Part model, mm, in its own coordinate system. A direction names the side the tool comes from. Round coordinates to 2 decimals unless told otherwise and drop trailing zeros. Write each loop counter-clockwise with the first axis right and the second up, starting at its lowest first coordinate (ties: lowest second). Pieces come first, ordered by that corner, then holes. Notation, with made-up numbers: M 60,39 L 66,39 A33 ccw 66,72 Z; hole C -20.5,89 d8. An arc over 180 degrees is marked long. Use one line per item in the form item = value. Start each with the question number.
Item 1: Mould opens along Y. For faces 5 (the face through (-15, 0, 20)), 6 (the face through (20, 10, 20)), 7 (the face through (14.141, 2.797, 20.07)) say: +Y half, -Y half, draft (parallel to the pull), parting line (faces both ways), or undercut.
Item 2: Cut at D-D, the plane z = 34. Give the cut face in (x, y), then the cut area to 3 significant figures.
Item 3: Flat gauge pins, fed straight in: pin 1 Ø5.5 at (x, z) = (-12.5, 23.5) entering from -Y; pin 2 Ø5.5 at (x, z) = (10.5, 23.5) entering from -Y; pin 3 Ø1.5 at (x, z) = (18, 17.5) entering from -Y. Where does each tip first touch, or does it go through?
Item 4: Cut at C-C, the plane y = 11.25. Give the cut face in (x, z), then the cut area to 3 significant figures.
Item 5: Cut at A-A, the plane x = -17. Give the cut face in (y, z), then the cut area to 3 significant figures.
Item 6: Which spindle directions (+Z, -Z, +X, -X, +Y, -Y) get a long thin tool onto all of the face, cutting with end or side? Do faces 1 (the face through (-11, 15, 20)), 2 (the face through (18, 4, 20)), 3 (the face through (-14, 20, 20)), 4 (the face through (8, 17, 20)). Say none if no direction does.
Item 7: Probe L1, parallel to Z at x = 18, y = 3.25; L2, parallel to Y at x = -8.5, z = 23.5; L3, parallel to X at y = 12.75, z = 23.5. List the from-to ranges inside material, lowest first.
Item 8: Cut at B-B, the plane z = 21.5. Give the cut face in (x, y), then the cut area to 3 significant figures.
from build123d import *

# Parameters (mm, degrees)
BOSS_EXTRUDE1_DEPTH     = 40
BOSS_EXTRUDE2_DEPTH     = 15
SKETCH9_R               = 3
BOSS_EXTRUDE3_DEPTH     = 40
CUT_EXTRUDE2_DEPTH      = 10
F_4_0_MM_DOWEL_HOLES2_D = 4


with BuildPart() as part:
    # Sketch2 → Boss-Extrude1 (new body)
    with BuildSketch(Plane.XY):
        Polygon((-20, 20), (-8, 20), (-8, 15), (-15, 15), (-15, 10), (15, 10), (15, 15), (8, 15), (8, 20), (20, 20), (20, 0), (-20, 0), align=None)
    extrude(amount=BOSS_EXTRUDE1_DEPTH)

    # Sketch3 → Boss-Extrude2 (add)
    with BuildSketch(Plane(origin=(0, 0, 0), x_dir=(-1, 0, 0), z_dir=(0, 0, -1))):
        with BuildLine():
            Line((-20, 0), (-14, 0))
            ThreePointArc((-14, 0), (-17, -3), (-20, 0))
        make_face()
    boss_extrude2 = extrude(amount=-BOSS_EXTRUDE2_DEPTH)

    # Mirror1: Boss-Extrude2 across plane
    add(boss_extrude2.mirror(Plane(origin=(0, 0, 20), x_dir=(1, 0, 0), z_dir=(0, 0, -1))))

    # Sketch9 → Boss-Extrude3 (add)
    with BuildSketch(Plane(origin=(0, 0, 0), x_dir=(-1, 0, 0), z_dir=(0, 0, -1))):
        with Locations((17, 0)):
            Circle(SKETCH9_R)
    extrude(amount=-BOSS_EXTRUDE3_DEPTH)

    # Sketch10 → Cut-Extrude2 (cut)
    with BuildSketch(Plane(origin=(0, 0, 25), x_dir=(-1, 0, 0), z_dir=(0, 0, -1))):
        with BuildLine():
            Line((-17, 4), (-20, 4))
            Line((-20, 4), (-20, 2.645751311))
            ThreePointArc((-20, 2.645751311), (-15.354248689, -3.645751311), (-17, 4))
        make_face()
    extrude(amount=CUT_EXTRUDE2_DEPTH, mode=Mode.SUBTRACT)

    # Ø4.0 mm Dowel Holes2 (through all)
    with Locations(Plane(origin=(0, 0, 0), x_dir=(-1, 0, 0), z_dir=(0, 0, -1))):
        with Locations((-17, 0)):
            f_4_0_mm_dowel_holes2 = Hole(F_4_0_MM_DOWEL_HOLES2_D / 2)

    # Mirror5: Ø4.0 mm Dowel Holes2 across plane
    add(f_4_0_mm_dowel_holes2.mirror(Plane.ZY), mode=Mode.SUBTRACT)


solid = part.part
Model answer:
q1.face_5 = undercut
q1.face_6 = draft
q1.face_7 = -Y half
q2.outline = M -20,0 A3 ccw -14,0 L 14,0 A3 ccw 20,0 L 20,20 L 8,20 L 8,15 L 15,15 L 15,10 L -15,10 L -15,15 L -8,15 L -8,20 L -20,20 Z; hole C -17,0 d4; hole C 17,0 d4
q2.area = 573 mm²
q3.pin_1 = -2.44
q3.pin_2 = 0
q3.pin_3 = 4
q4.outline = M -20,0 L -15,0 L -15,40 L -20,40 Z; M 15,0 L 20,0 L 20,40 L 15,40 Z
q4.area = 400 mm²
q5.outline = M -3,0 L -2,0 L -2,40 L -3,40 Z; M 2,0 L 20,0 L 20,40 L 2,40 Z
q5.area = 760 mm²
q6.face_1 = +Z, -Z
q6.face_2 = +X, -Y
q6.face_3 = +Z, -Z, +X, -X, +Y
q6.face_4 = +Z, -Z, +Y
q7.L1 = 0 to 15, 25 to 40
q7.L2 = 0 to 10, 15 to 20
q7.L3 = -20 to -15, 15 to 20
q8.outline = M -20,0 A3 ccw -14,0 L 13,0 A4 cw 17,4 L 20,4 L 20,20 L 8,20 L 8,15 L 15,15 L 15,10 L -15,10 L -15,15 L -8,15 L -8,20 L -20,20 Z; hole C -17,0 d4
q8.area = 547 mm²
